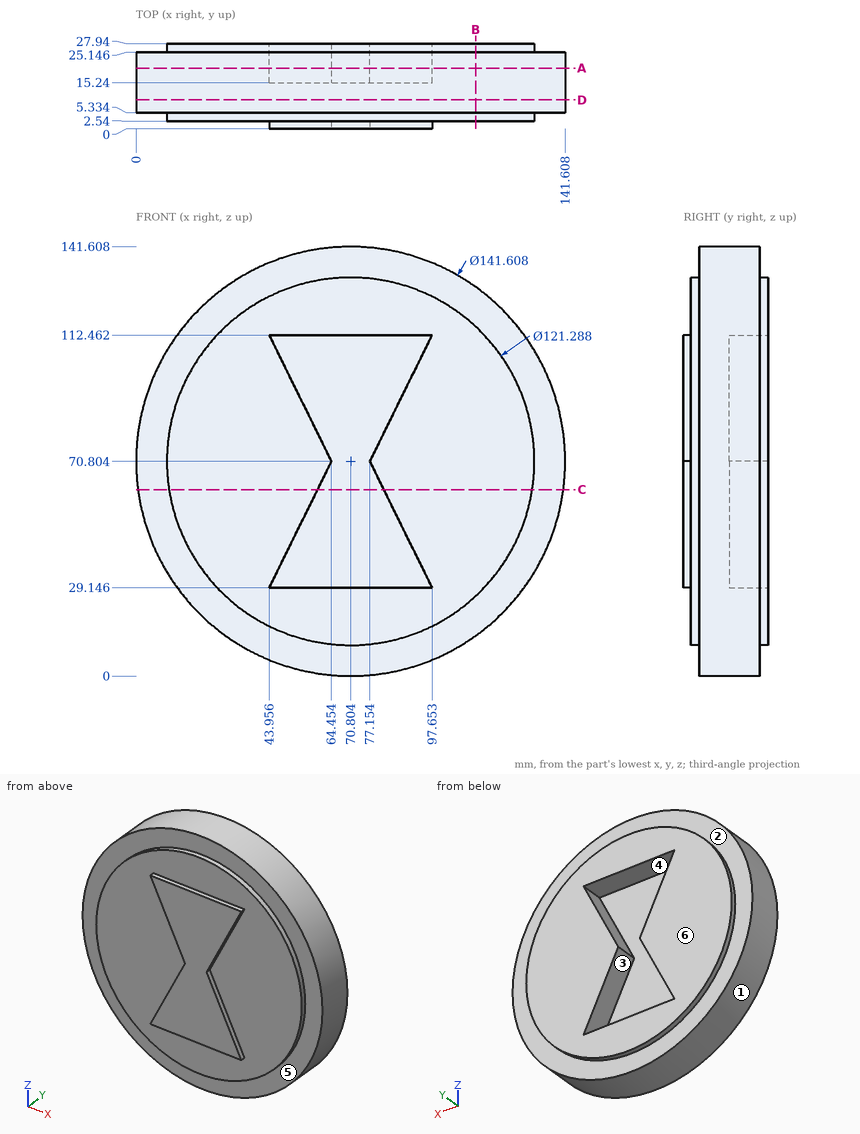
Geometry: see drawing. Coordinates: mm, zero at the bounding-box minimum. A direction names the side the tool comes from. Round coordinates to 2 decimals unless told otherwise and drop trailing zeros. Order: outer loops, then holes, each group sorted by start corner. A loop starts at its lowest first (then second) coordinate and runs counter-clockwise, first axis right, second up. Notation, with made-up numbers: (28.25, 28) - (79.25, 28) arc R12 cw to (79.25, 47) - close; hole circle Ø7 at (-23, 41.5). An arc over 180 degrees is marked (long way). Use a Markdown table: item, result. Add a question column.
1. First-contact query: pin 1 (1.5 mm diameter, centred on x = 79.5, y = 24.5, fed in from -Z); pin 2 (3 mm diameter, centred on x = 68, z = 74, fed in from +Y); pin 3 (10 mm diameter, centred on x = 80.5, y = 21.5, fed in from +Z). Flat tips, straight axial feed; report the tip coordinate or a pass-through.
2. Section query B-B (x = 112). Return the cut outline in (y, z).
3. Section query C-C (z = 61.5). Return the cut outline in (x, y) (1 decimal), then the cut area to 3 significant figures.
4. Line query: probe 1 along Y at (x, z) = (70, 10.5); probe 2 along X at (y, z) = (3, 71); probe 3 along Y at (x, z) = (123, 116). Output: solid intervals per line, ascending.
5. Mould query, pull axis X, two halves, no side actions, for the marked faces 1, 2 and 3. Classes: +X half, -X half, draft (parallel to the pull), parting line (faces both ways), or undercut.
6. Section query D-D (y = 9.5). Return the cut outline in (x, z).
7. Set-up query: the marked faces 4, 5 and 6. Return all of +Z, -Z, +X, -X, +Y, -Y with unobstructed straight access to the full face (end or side cutting, diameter ignored); none if empty.
8. Section query A-A (y = 20). Return the cut outline in (x, z) (1 decimal), then the cut area to 3 significant figures.
Derived:
| question | item | result |
|---|---|---|
| 1 | pin 1 | z = 0.45 |
| 1 | pin 2 | y = 15.24 |
| 1 | pin 3 | z = 141.45 |
| 2 | outline | (2.54, 26.3) - (5.33, 26.3) - (5.33, 13.22) - (25.15, 13.22) - (25.15, 26.3) - (27.94, 26.3) - (27.94, 115.31) - (25.15, 115.31) - (25.15, 128.39) - (5.33, 128.39) - (5.33, 115.31) - (2.54, 115.31) - close |
| 3 | outline | (0.6, 5.3) - (10.9, 5.3) - (10.9, 2.5) - (59.9, 2.5) - (59.9, 0) - (81.7, 0) - (81.7, 2.5) - (130.7, 2.5) - (130.7, 5.3) - (141, 5.3) - (141, 25.1) - (130.7, 25.1) - (130.7, 27.9) - (81.7, 27.9) - (81.7, 15.2) - (59.9, 15.2) - (59.9, 27.9) - (10.9, 27.9) - (10.9, 25.1) - (0.6, 25.1) - close |
| 3 | area | 3,230 mm2 |
| 4 | probe 1 | 2.54 to 27.94 |
| 4 | probe 2 | 10.16 to 131.45 |
| 4 | probe 3 | 5.33 to 25.15 |
| 5 | face 1 | parting line |
| 5 | face 2 | draft |
| 5 | face 3 | undercut |
| 6 | outline | circle Ø141.61 at (70.8, 70.8) |
| 7 | face 4 | +Y |
| 7 | face 5 | -Y |
| 7 | face 6 | +Z, -Z, +X, -X, +Y |
| 8 | outline | circle Ø141.6 at (70.8, 70.8); hole (44, 29.1) - (97.7, 29.1) - (77.2, 70.8) - (97.7, 112.5) - (44, 112.5) - (64.5, 70.8) - close |
| 8 | area | 13,000 mm2 |
